Can you work these out from the model? Positions are in its coordinate system, mm. A direction names the side the tool comes from. Coordinates: 2 decimals unless noted, no trailing zeros. Order: outer loops, then holes, each group sorted by start corner. A loop starts at its lowest first (then second) coordinate and runs counter-clockwise, first axis right, second up. Notation, with made-up numbers: (2.5, 72.25) -> (15.5, 72.25) arc R19 ccw to (15.5, 77.25) -> close; hole circle Ø5 at (52.5, 15.25). An arc over 180 degrees is marked (long way). Answer as a JSON object with one key per item and string values. Group by question number.
(1) I want a section at C-C, the plane z = -7.5. List the corners of the cut face in (x, y) for me, plus the area to 3 significant figures.
(2) Which directions (+Z, -Z, +X, -X, +Y, -Y) give clear straight access to the entire face, cutting with the end or side of a thin tool? Please do faces 1 (the flat face through (1, 0.2, -4)), 2 (the flat face through (1, 13.2, -4)), 3 (the flat face through (0, 5, -4)), 4 (the flat face through (1.2, 11, -1)), 5 (the flat face through (-0.2, 24, -1)).
(3) If we mould it in two halves opening along Y, with no side actions, what happens to faces 6 (the flat face through (1, 22.4, -4)), 7 (the flat face through (2, 11, -1)), 8 (the flat face through (1, 9.4, -4))? For each: pulls with the +Y half, pulls with the -Y half, needs draft (parallel to the pull), parting line crosses it, or undercut.
(4) I want a section at D-D, the plane y = 17.8. List the corners of the cut face in (x, z) for me.
(5) I want a section at A-A, the plane x = 0.5. List the corners of the cut face in (y, z) for me.
(6) I want a section at B-B, the plane z = -1.5. List the corners of the cut face in (x, y) for me, plus the area to 3 significant figures.
(7) For pin 1 (1.1 mm diameter, centred on x = 0.5, z = -5.5, fed in from -Y); pin 2 (1 mm diameter, centred on y = -0.5, z = -1, fed in from +X); pin 3 (2 mm diameter, centred on x = -0.5, y = 10.5, fed in from -Z), each with a flat end and sliding along its axis, tell me the tip position at first contact or that it passes through.
(8) I need wall thicknesses on line 1 (X direction, y = 10, z = -1); line 2 (Y direction, x = 0.35, z = -2); line 3 (Y direction, x = 1.15, z = -7.5). Which ranges of each line are inside material? Lowest first, please.
Autodesk Inventor part; units mm, degrees
ref_plane "YZ Plane" through (0, 0, 0) normal (1, 0, 0) x (0, 1, 0)
ref_plane "XZ Plane" through (0, 0, 0) normal (0, 1, 0) x (-1, 0, 0)
ref_plane "XY Plane" through (0, 0, 0) normal (0, 0, 1) x (1, 0, 0)
sketch "Sketch1" plane through (0, 0, 0) normal (0, 0, 1) x (1, 0, 0)
  line L0 (0, 0) -> (0, -2.7)
  line L1 (0, -2.7) -> (-2.5, -2.7)
  line L2 (-2.5, -2.7) -> (-2.5, 25.3)
  line L3 (0, 25.3) -> (-2.5, 25.3)
  line L4 (0, 25.3) -> (0, 22.6)
  line L5 (0, 22.6) -> (2, 22.6)
  line L6 (2, 27.3) -> (2, 22.6)
  line L7 (-4.5, 27.3) -> (2, 27.3)
  line L8 (-4.5, -4.7) -> (-4.5, 27.3)
  line L9 (-4.5, -4.7) -> (2, -4.7)
  line L10 (2, 0) -> (2, -4.7)
  line L11 (0, 0) -> (2, 0)
  line L12 (-0.2, 25.1) -> (-2.55, 25.1)
  line L13 (-2.55, 25.1) -> (-2.55, -2.5)
  line L14 (-2.55, -2.5) -> (-0.2, -2.5)
  line L15 (-0.2, -2.5) -> (-0.2, 25.1)
  line L16 (0, 22.6) -> (0, 22.4) construction
  line L17 (1, 13) -> (2, 13)
  line L18 (1, 9.6) -> (1, 13)
  line L19 (2, 9.6) -> (1, 9.6)
  line L20 (2, 13) -> (2, 9.6)
  line L21 (1, 11.3) -> (1.2, 11.3) construction
  line L22 (2, 13) -> (1.2, 13)
  line L23 (1.2, 13) -> (1.2, 9.6)
  line L24 (1.2, 9.6) -> (2, 9.6)
  line L25 (2, 9.6) -> (2, 13)
  line L26 (1.2, 13) -> (1.2, 13.2)
  line L27 (2, 13.2) -> (-0.2, 13.2)
  line L28 (-0.2, 13.2) -> (-0.2, 22.4)
  line L29 (-0.2, 22.4) -> (2, 22.4)
  line L30 (2, 22.4) -> (2, 13.2)
  line L31 (2, 13.2) -> (2, 13)
  line L32 (2, 9.6) -> (1.2, 9.6)
  line L33 (1.2, 9.6) -> (1.2, 9.4)
  line L34 (1.2, 9.4) -> (2, 9.4)
  line L35 (2, 9.4) -> (2, 9.6)
  line L36 (2, 9.4) -> (-0.2, 9.4)
  line L37 (-0.2, 9.4) -> (-0.2, 0.2)
  line L38 (-0.2, 0.2) -> (2, 0.2)
  line L39 (2, 0.2) -> (2, 9.4)
  point P0 (-1.25, 11.3)
  point P1 (-1.25, 11.3)
  dimension "d0" = 2.35
  dimension "d1" = 27.6
  dimension "d2" = 0.2
  dimension "d3" = 0.2
  dimension "d4" = 0.2
  dimension "d5" = 0.2
  dimension "d6" = 9.2
extrude "Extrusion1" add sketch "Sketch1" against normal blind 2 contours L14 L13 L12 L2 | L2 L12 L15 L14 | L15 L36 L34 L39 L38 | L29 L30 L27 L15 | L33 L19 L35 L34 | L27 L31 L17 L26 | L23 L17 L20 L19
sketch "Sketch2" plane through (2, 0.2, 0) normal (1, 0, 0) x (0, 0, -1)
  arc A0 (9, -0.2) -> (9, 9.4) centre (9, 4.6) ccw
  arc A1 (9, 12.8) -> (9, 22.4) centre (9, 17.6) ccw
  circle A2 centre (9, 4.6) radius 4.6
  circle A3 centre (9, 17.6) radius 4.6
  line L0 (2, 22.2) -> (2, 0)
  line L1 (9, 0) -> (2, 0)
  line L2 (9, 9.2) -> (2, 9.2)
  line L3 (2, 0) -> (2, 9.2)
  line L4 (9, 13) -> (2, 13)
  line L5 (2, 13) -> (2, 22.2)
  line L6 (0, 22.2) -> (2, 22.2)
  line L7 (9, 22.2) -> (2, 22.2)
  point P0 (0, -0.2)
  dimension "d12" = 9.2
  dimension "d13" = 9.2
extrude "Extrusion3" add sketch "Sketch2" against normal blind 2 contours L0 L7 A3 L4 | A2 L1 L0 L2
properties part number "prototype7_2_3DPrint"
Computed values:
{
 "1": {"outline": "(0, 0.2) -> (2, 0.2) -> (2, 0.45) -> (0, 0.45) -> close; (0, 9.15) -> (2, 9.15) -> (2, 9.4) -> (0, 9.4) -> close; (0, 13.2) -> (2, 13.2) -> (2, 13.45) -> (0, 13.45) -> close; (0, 22.15) -> (2, 22.15) -> (2, 22.4) -> (0, 22.4) -> close", "area": "2.01 mm2"},
 "2": {"face 1": "+Z, -Z, +X, -Y", "face 2": "-Z", "face 3": "-Z, -X, +Y, -Y", "face 4": "+Z, -Z", "face 5": "+Z, -Z, +X, +Y"},
 "3": {"face 6": "pulls with the +Y half", "face 7": "needs draft", "face 8": "undercut"},
 "4": {"outline": "(-2.55, -2) -> (0, -2) -> (0, -4.4) -> (2, -4.4) -> (2, 0) -> (-2.55, 0) -> close"},
 "5": {"outline": "(0.2, -9) arc R4.6 cw to (9.4, -9) -> (9.4, 0) -> (0.2, 0) -> close; (13.2, -9) arc R4.6 cw to (22.4, -9) -> (22.4, 0) -> (13.2, 0) -> close"},
 "6": {"outline": "(-2.55, -2.5) -> (-0.2, -2.5) -> (-0.2, 0.2) -> (2, 0.2) -> (2, 22.4) -> (-0.2, 22.4) -> (-0.2, 25.1) -> (-2.55, 25.1) -> close; hole (-0.2, 9.4) -> (1.2, 9.4) -> (1.2, 13.2) -> (-0.2, 13.2) -> close", "area": "108 mm2"},
 "7": {"pin 1": "stops at y = 0.2", "pin 2": "stops at x = -0.2", "pin 3": "stops at z = -2"},
 "8": {"line 1": "x = -2.55 to -0.2, 1.2 to 2", "line 2": "y = 0.2 to 9.4, 13.2 to 22.4", "line 3": "y = 0.2 to 0.45, 9.15 to 9.4, 13.2 to 13.45, 22.15 to 22.4"}
}
